from build123d import *

# Parameters (mm, degrees)
SKETCH1_R           = 1.85
SKETCH1_R_2         = 2.1
SKETCH1_R_3         = 3.175
BOSS_EXTRUDE1_DEPTH = 4.3


with BuildPart() as part:
    # Sketch1 → Boss-Extrude1 (new body)
    with BuildSketch(Plane(origin=(0, 0, 0), x_dir=(1, 0, 0), z_dir=(0, 1, 0))):
        with BuildLine():
            Line((-143.318, 44.044009042), (143.318, 44.044009042))
            ThreePointArc((143.318, 44.044009042), (146.853533906, 42.579542947), (148.318, 39.044009042))
            Line((148.318, 39.044009042), (148.318, -177.955990958))
            ThreePointArc((148.318, -177.955990958), (146.853533906, -181.491524864), (143.318, -182.955990958))
            Line((143.318, -182.955990958), (111, -182.955990958))
            Line((111, -182.955990958), (111, -214.955990958))
            Line((111, -214.955990958), (76, -214.955990958))
            ThreePointArc((76, -214.955990958), (72.464466094, -213.491524864), (71, -209.955990958))
            Line((71, -209.955990958), (71, -183.438106878))
            ThreePointArc((71, -183.438106878), (70.090326299, -180.562479856), (67.692307692, -178.733205745))
            ThreePointArc((67.692307692, -178.733205745), (0, -166.929251079), (-67.692307692, -178.733205745))
            ThreePointArc((-67.692307692, -178.733205745), (-70.090326299, -180.562479856), (-71, -183.438106878))
            Line((-71, -183.438106878), (-71, -209.955990958))
            ThreePointArc((-71, -209.955990958), (-72.464466094, -213.491524864), (-76, -214.955990958))
            Line((-76, -214.955990958), (-111, -214.955990958))
            Line((-111, -214.955990958), (-111, -182.955990958))
            Line((-111, -182.955990958), (-143.318, -182.955990958))
            ThreePointArc((-143.318, -182.955990958), (-146.853533906, -181.491524864), (-148.318, -177.955990958))
            Line((-148.318, -177.955990958), (-148.318, 39.044009042))
            ThreePointArc((-148.318, 39.044009042), (-146.853533906, 42.579542947), (-143.318, 44.044009042))
        make_face()
        with Locations((126, 26.544009042)):
            Circle(SKETCH1_R, mode=Mode.SUBTRACT)
        with Locations((134, 18.544009042)):
            Circle(SKETCH1_R, mode=Mode.SUBTRACT)
        with Locations((126, 10.544009042)):
            Circle(SKETCH1_R, mode=Mode.SUBTRACT)
        with Locations((107.318, -7.955990958)):
            Circle(SKETCH1_R_2, mode=Mode.SUBTRACT)
        with Locations((107.318, 24.044009042)):
            Circle(SKETCH1_R_2, mode=Mode.SUBTRACT)
        with Locations((18.318, 23.544009041)):
            Circle(SKETCH1_R_2, mode=Mode.SUBTRACT)
        with Locations((27.318, 24.044009042)):
            Circle(SKETCH1_R_2, mode=Mode.SUBTRACT)
        with Locations((18.318, -8.455990959)):
            Circle(SKETCH1_R_2, mode=Mode.SUBTRACT)
        with Locations((27.318, -7.955990958)):
            Circle(SKETCH1_R_2, mode=Mode.SUBTRACT)
        with Locations((-134, 18.544009042)):
            Circle(SKETCH1_R, mode=Mode.SUBTRACT)
        with Locations((-126, 10.544009042)):
            Circle(SKETCH1_R, mode=Mode.SUBTRACT)
        with Locations((-126, 26.544009042)):
            Circle(SKETCH1_R, mode=Mode.SUBTRACT)
        with Locations((-45.682, -8.455990959)):
            Circle(SKETCH1_R_2, mode=Mode.SUBTRACT)
        with Locations((-45.682, 23.544009041)):
            Circle(SKETCH1_R_2, mode=Mode.SUBTRACT)
        with Locations((-43.68216529, -145.455990959)):
            Circle(SKETCH1_R_2, mode=Mode.SUBTRACT)
        with Locations((-43.68216529, -81.455495942)):
            Circle(SKETCH1_R_2, mode=Mode.SUBTRACT)
        with Locations((44.318, -145.455990959)):
            Circle(SKETCH1_R_2, mode=Mode.SUBTRACT)
        with Locations((44.318, -113.455990958)):
            Circle(SKETCH1_R_2, mode=Mode.SUBTRACT)
        with Locations((44.318, -81.455495942)):
            Circle(SKETCH1_R_2, mode=Mode.SUBTRACT)
        with Locations((-96, -191.955990958)):
            Circle(SKETCH1_R, mode=Mode.SUBTRACT)
        with Locations((-104, -199.955990958)):
            Circle(SKETCH1_R, mode=Mode.SUBTRACT)
        with Locations((-88, -199.955990958)):
            Circle(SKETCH1_R, mode=Mode.SUBTRACT)
        with Locations((-96, -207.955990958)):
            Circle(SKETCH1_R, mode=Mode.SUBTRACT)
        with Locations((96, -207.955990958)):
            Circle(SKETCH1_R, mode=Mode.SUBTRACT)
        with Locations((96, -191.955990958)):
            Circle(SKETCH1_R, mode=Mode.SUBTRACT)
        with Locations((104, -199.955990958)):
            Circle(SKETCH1_R, mode=Mode.SUBTRACT)
        with Locations((88, -199.955990958)):
            Circle(SKETCH1_R, mode=Mode.SUBTRACT)
        with Locations((124.318, -81.455495942)):
            Circle(SKETCH1_R_2, mode=Mode.SUBTRACT)
        with Locations((124.318, -113.455495942)):
            Circle(SKETCH1_R_2, mode=Mode.SUBTRACT)
        with Locations((-52.68216529, -129.955990958)):
            Circle(SKETCH1_R_3, mode=Mode.SUBTRACT)
        with Locations((-107.68216529, -129.955990958)):
            Circle(SKETCH1_R_3, mode=Mode.SUBTRACT)
    extrude(amount=BOSS_EXTRUDE1_DEPTH)


solid = part.part
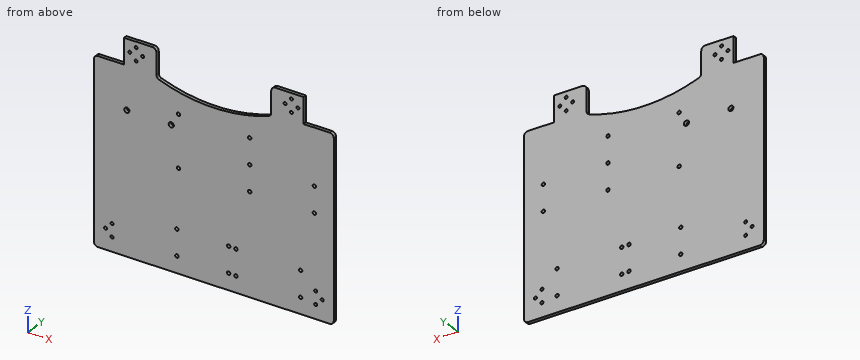
Work out the finished part from the listing and answer in its coordinate system (mm). Round coordinates to 2 decimals unless told otherwise and drop trailing zeros. Loops run counter-clockwise (first coordinate to the right, second up) from the corner with the lowest first, then second, coordinate; pieces in that order, holes last. Notation, with made-up numbers: (-3.5, 79.5) -> (41.5, 79.5) arc R21 ccw to (41.5, 106.5) -> close; hole circle Ø3 at (-39, 68.25). An arc over 180 degrees is marked (long way). Use one line per item in the form item = value.
(1) Flat-ended cylindrical pins translate along their axes: P1, Ø2, axis at y = 1.5, z = 199.5, coming from the -X side; P2, Ø1, axis at x = -23, y = 3.5, coming from the +Z side. Find the tip coordinate at first contact, or state that the pin passes through.
Answer list:
P1 = -111
P2 = 168.31
(2) Find section C-C on y = 2.15. Give the number of separate pieces and of enclosed holes in the cut face, then the cut area to 3 significant figures.
Answer list:
separate_pieces = 1
enclosed_holes = 31
area = 67,800 mm2
(3) Find section A-A on z = 171.5. Give the vertices of the cut face in (x, y).
Answer list:
outline = (-148.32, 0) -> (-42.51, 0) -> (-42.51, 4.3) -> (-148.32, 4.3) -> close; (42.51, 0) -> (148.32, 0) -> (148.32, 4.3) -> (42.51, 4.3) -> close
(4) Find section B-B on x = 9.5. Give the vertices of the cut face in (y, z) (3 decimals).
Answer list:
outline = (0, -44.044) -> (4.3, -44.044) -> (4.3, 167.155) -> (0, 167.155) -> close
(5) Straight lines are drawn through the part: line 1 (Z direction, x = -126, y = 1.1); line 2 (X direction, y = 1.6, z = 200); line 3 (Z direction, x = 96, y = 1.65). For each, find the intervals that lie inside material, in ascending order.
Answer list:
line_1 = -44.04 to -28.39, -24.69 to -12.39, -8.69 to 182.96
line_2 = -111 to -105.85, -102.15 to -89.85, -86.15 to -71, 71 to 86.15, 89.85 to 102.15, 105.85 to 111
line_3 = -44.04 to 190.11, 193.81 to 206.11, 209.81 to 214.96
